Autodesk Inventor part; units mm, degrees
ref_plane "YZ Plane" through (0, 0, 0) normal (1, 0, 0) x (0, 1, 0)
ref_plane "XZ Plane" through (0, 0, 0) normal (0, 1, 0) x (-1, 0, 0)
ref_plane "XY Plane" through (0, 0, 0) normal (0, 0, 1) x (1, 0, 0)
sketch "Sketch1" plane through (0, 0, 0) normal (0, 1, 0) x (-1, 0, 0)
  line L0 (0, 0) -> (93.98, 0)
  line L1 (93.98, 0) -> (93.98, -93.98)
  line L2 (93.98, -93.98) -> (0, -93.98)
  line L3 (0, -93.98) -> (0, 0)
  line L4 (0, -93.98) -> (12.7, -93.98)
  line L5 (93.98, -93.98) -> (81.28, -93.98)
  line L6 (12.7, -93.98) -> (78.74, -93.98)
  line L7 (12.7, -93.98) -> (81.28, -93.98)
  arc A0 (33.54, -38.745) -> (29.94, -38.745) centre (31.74, -38.745) ccw
  circle A1 centre (31.74, -38.745) radius 1.8
  arc A2 (29.94, -8.245) -> (33.54, -8.245) centre (31.74, -8.245) ccw
  circle A3 centre (31.74, -8.245) radius 1.8
  arc A4 (64.04, -38.745) -> (60.44, -38.745) centre (62.24, -38.745) ccw
  circle A5 centre (62.24, -38.745) radius 1.8
  arc A6 (60.44, -8.245) -> (64.04, -8.245) centre (62.24, -8.245) ccw
  circle A7 centre (62.24, -8.245) radius 1.8
  line L8 (0, -93.98) -> (12.7, -93.98)
  line L9 (93.98, -93.98) -> (81.28, -93.98)
  line L10 (0, 0) -> (0, -46.99)
  line L11 (0, -46.99) -> (0, -93.98)
  circle A8 centre (60.49, -56.985) radius 1.75
  circle A9 centre (60.49, -83.985) radius 1.75
  circle A10 centre (33.49, -56.985) radius 1.75
  circle A11 centre (33.49, -83.985) radius 1.75
extrude "Extrusion5" add sketch "Sketch1" along normal blind 1.5875
fillet "Fillet2" radius 3.175 4 edges at (0, 0.7937, 0) (0, 0.7937, -93.98) (-93.98, 0.7937, 0) (-93.98, 0.7937, -93.98)
sketch "Sketch4" plane through (0, 1.5875, 0) normal (0, 1, 0) x (1, 0, 0)
  line L0 (-3.175, 93.98) -> (-90.805, 93.98)
  circle A0 centre (-88.9, 5.08) radius 1.75
  circle A1 centre (-88.9, 88.9) radius 1.75
  circle A2 centre (-5.08, 5.08) radius 1.75
  circle A3 centre (-5.08, 88.9) radius 1.75
  point P0 (0, 0)
  dimension "d37" = 3.5
  dimension "d38" = 3.5
  dimension "d39" = 3.5
  dimension "d40" = 3.5
extrude "Extrusion6" cut sketch "Sketch4" against normal blind 1.5875
properties part number "bottomPlate"
Read the model definition and answer for the solid it produces. Units are mm, in the model's axes. Round coordinates to 2 decimals unless told otherwise and drop trailing zeros. Write each loop counter-clockwise with the first axis right and the second up, starting at its lowest first coordinate (ties: lowest second). Pieces come first, ordered by that corner, then holes. Notation, with made-up numbers: (20.5, -26) - (76.5, -26) arc R22 cw to (76.5, 9) - close; hole circle Ø6 at (43, -16). An arc over 180 degrees is marked (long way). One line per item, written item: value.
Q1. Find section A-A (z = -88.9). Determine the outline of the cut face in (x, y), and give its area (3 significant figures).
The answers:
outline: (-93.98, 0) - (-90.65, 0) - (-90.65, 1.59) - (-93.98, 1.59) - close; (-87.15, 0) - (-6.83, 0) - (-6.83, 1.59) - (-87.15, 1.59) - close; (-3.33, 0) - (0, 0) - (0, 1.59) - (-3.33, 1.59) - close
area: 138 mm2
Q2. Find section B-B (x = -5.08). Determine the outline of the cut face in (y, z), and give its area (3 significant figures).
The answers:
outline: (0, -93.98) - (1.59, -93.98) - (1.59, -90.65) - (0, -90.65) - close; (0, -87.15) - (1.59, -87.15) - (1.59, -6.83) - (0, -6.83) - close; (0, -3.33) - (1.59, -3.33) - (1.59, 0) - (0, 0) - close
area: 138 mm2
Q3. This flat-tipped pin is pushed along its axis until it touches: P1, Ø4.5, axis at x = -62.24, z = -38.745, coming from the -Y side. Where does it stop, or does it pass through?
The answers:
P1: stops at y = 0
Q4. For a pull along Z with two mould halves and no side action, classify faces 1 (the cylindrical face through (-0.95, 0.8, -0.91)), 2 (the cylindrical face through (-34.298, 0.783, -82.432)), 3 (the cylindrical face through (-93, 0.8, -93.1)) as pulls with the +Z half, pulls with the -Z half, needs draft (parallel to the pull), parting line crosses it, or undercut.
The answers:
face 1: pulls with the +Z half
face 2: undercut
face 3: pulls with the -Z half
Q5. Straight lines are drawn through the part: line 1 (X direction, y = 1.25, z = -8); line 2 (Z direction, x = -88.9, y = 0.7). For each, find the intervals that lie inside material, in ascending order. Write a range as from..to.
The answers:
line 1: x = -93.98..-64.02, -60.46..-33.52, -29.96..0
line 2: z = -93.98..-90.65, -87.15..-6.83, -3.33..0
